```python
from build123d import *

# Parameters (mm, degrees)
SKETCH_R        = 1.56961
SKETCH_R_2      = 11.5
PAD_DEPTH       = 50
POCKET_DEPTH    = 45
SKETCH002_W     = 4.8693872445
SKETCH002_H     = 8
POCKET001_DEPTH = 5


with BuildPart() as part:
    # Sketch → Pad (new body)
    with BuildSketch(Plane.XY):
        with BuildLine():
            Line((-26.5555397501, 36.4599848379), (26.5555397501, 36.4599848379))
            ThreePointArc((36.4599848378, 26.5555397501), (33.5590400355, 33.5590400355), (26.5555397501, 36.4599848378))
            Line((36.4599848379, 26.5555397501), (36.4599848379, -26.5555397501))
            ThreePointArc((26.5555397501, -36.4599848378), (33.5590400355, -33.5590400355), (36.4599848378, -26.5555397501))
            Line((26.5555397501, -36.4599848379), (-26.5555397501, -36.4599848379))
            ThreePointArc((-36.4599848378, -26.5555397501), (-33.5590400355, -33.5590400355), (-26.5555397501, -36.4599848378))
            Line((-36.4599848379, -26.5555397501), (-36.4599848379, 26.5555397501))
            ThreePointArc((-26.5555397501, 36.4599848378), (-33.5590400355, 33.5590400355), (-36.4599848378, 26.5555397501))
        make_face()
        with Locations((15.5, 15.5)):
            Circle(SKETCH_R, mode=Mode.SUBTRACT)
        with Locations((-15.5, 15.5)):
            Circle(SKETCH_R, mode=Mode.SUBTRACT)
        with Locations((15.5, -15.5)):
            Circle(SKETCH_R, mode=Mode.SUBTRACT)
        with Locations((-15.5, -15.5)):
            Circle(SKETCH_R, mode=Mode.SUBTRACT)
        Circle(SKETCH_R_2, mode=Mode.SUBTRACT)
    extrude(amount=PAD_DEPTH)

    # Sketch001 → Pocket (cut)
    with BuildSketch(Plane(origin=(0, 0, 0), x_dir=(1, 0, 0), z_dir=(0, 0, -1))):
        with BuildLine():
            Line((-21.2160363943, 31.5905975933), (21.2160363942, 31.5905975933))
            ThreePointArc((31.5905975933, 21.2160363942), (28.55195897, 28.55195897), (21.2160363942, 31.5905975933))
            Line((31.5905975933, 21.2160363942), (31.5905975933, -21.2160363942))
            ThreePointArc((21.2160363943, -31.5905975933), (28.55195897, -28.5519589699), (31.5905975933, -21.2160363942))
            Line((21.2160363943, -31.5905975933), (-21.2160363943, -31.5905975933))
            ThreePointArc((-31.5905975933, -21.2160363943), (-28.5519589699, -28.55195897), (-21.2160363942, -31.5905975933))
            Line((-31.5905975933, -21.2160363943), (-31.5905975933, 21.2160363943))
            ThreePointArc((-21.2160363943, 31.5905975933), (-28.55195897, 28.55195897), (-31.5905975933, 21.2160363942))
        make_face()
    extrude(amount=-POCKET_DEPTH, mode=Mode.SUBTRACT)

    # Sketch002 → Pocket001 (cut)
    with BuildSketch(Plane(origin=(0, 0, 0), x_dir=(1, 0, 0), z_dir=(0, 0, -1))):
        with Locations((-34.0252912156, -0.0510141845)):
            Rectangle(SKETCH002_W, SKETCH002_H)
    extrude(amount=-POCKET001_DEPTH, mode=Mode.SUBTRACT)


solid = part.part
```
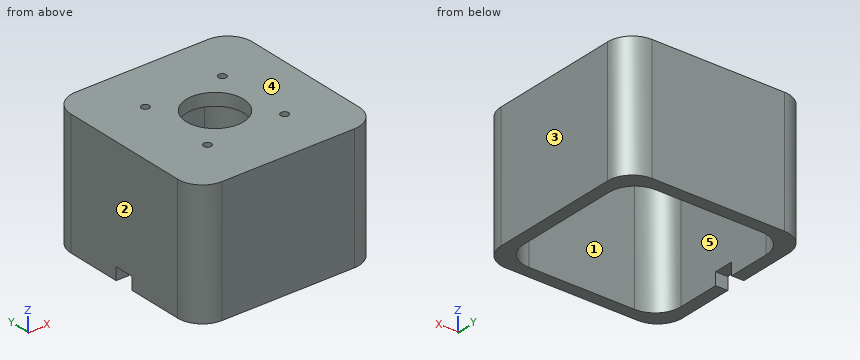
Input: part model. Units: mm. Frame: model coordinates. Face numbers are marked on the shaded views. A direction names the side the tool comes from. Give positions to 0.01 mm unless a question says otherwise; leave off trailing zeros. Loops run counter-clockwise (first coordinate to the right, second up) from the corner with the lowest first, then second, coordinate; pieces in that order, holes last.
1) Line query: L1, parallel to Y at x = -15.5, z = 48.7; L2, parallel to X at y = 12.5, z = 38. Output: solid intervals per line, ascending.
A:
L1: y = -36.46 to -17.07, -13.93 to 13.93, 17.07 to 36.46
L2: x = -36.46 to -31.59, 31.59 to 36.46
2) Contact query for flat-ended pins moving along their axis: pin 1 (5 mm diameter, centred on x = 2, y = -14.5, fed in from -Z); pin 2 (5.5 mm diameter, centred on x = -33, y = 0.5, fed in from -Z); pin 3 (5.5 mm diameter, centred on x = -34, z = 1.5, fed in from +Y). Output: stop coordinate, or through.
A:
pin 1: stops at z = 45
pin 2: stops at z = 5
pin 3: stops at y = 35.28
3) Section query B-B on y = 0. Return the cut outline in (x, z).
A:
outline: (-36.46, 5) - (-31.59, 5) - (-31.59, 45) - (-11.5, 45) - (-11.5, 50) - (-36.46, 50) - close; (11.5, 45) - (31.59, 45) - (31.59, 0) - (36.46, 0) - (36.46, 50) - (11.5, 50) - close
4) Mould query, pull axis X, two halves, no side actions, for the marked faces 3, 4 and 5. Classes: released by +X, released by -X, zero draft, split by the parting line, or undercut.
A:
face 3: released by +X
face 4: zero draft
face 5: undercut
5) Section query A-A on x = 15.5. Return the cut outline in (y, z).
A:
outline: (-36.46, 0) - (-31.59, 0) - (-31.59, 45) - (-17.07, 45) - (-17.07, 50) - (-36.46, 50) - close; (-13.93, 45) - (13.93, 45) - (13.93, 50) - (-13.93, 50) - close; (17.07, 45) - (31.59, 45) - (31.59, 0) - (36.46, 0) - (36.46, 50) - (17.07, 50) - close
6) Section query D-D on x = 0. Return the cut outline in (y, z), and give its area (3 significant figures).
A:
outline: (-36.46, 0) - (-31.59, 0) - (-31.59, 45) - (-11.5, 45) - (-11.5, 50) - (-36.46, 50) - close; (11.5, 45) - (31.59, 45) - (31.59, 0) - (36.46, 0) - (36.46, 50) - (11.5, 50) - close
area: 688 mm2
7) Reachability of the marked faces 1 and 2 from +Z, -Z, +X, -X, +Y, -Y: full face, straight path, thin tool, end or side. Return the list, or none.
A:
face 1: -Z
face 2: +Z, -Z, -X, +Y, -Y
